Autodesk Inventor part; units mm, degrees
ref_plane "YZ Plane" through (0, 0, 0) normal (1, 0, 0) x (0, 1, 0)
ref_plane "XZ Plane" through (0, 0, 0) normal (0, 1, 0) x (-1, 0, 0)
ref_plane "XY Plane" through (0, 0, 0) normal (0, 0, 1) x (1, 0, 0)
sketch "Sketch1" plane through (0, 0, 0) normal (0, 0, 1) x (1, 0, 0)
  circle A0 centre (0, 0) radius 28.575
  circle A1 centre (0, 0) radius 19.05
  dimension "d0" = 57.15
  dimension "d8" = 38.1
sketch "Sketch2" plane through (0, 0, 0) normal (0, 0, 1) x (1, 0, 0)
  circle A0 centre (0, 0) radius 23.8125
  circle A1 centre (0, 23.8125) radius 2.5908
  circle A2 centre (-20.6222, 11.9063) radius 2.5908
  circle A3 centre (-20.6222, -11.9062) radius 2.5908
  circle A4 centre (0, -23.8125) radius 2.5908
  circle A5 centre (20.6222, -11.9063) radius 2.5908
  circle A6 centre (20.6222, 11.9062) radius 2.5908
  dimension "d15" = 47.625
  dimension "d16" = 5.1816
  dimension "d19" = 360
extrude "Extrusion1" add sketch "Sketch1" along normal blind 13.97
extrude "Extrusion2" cut sketch "Sketch2" along normal blind 13.97 contours A6 A0 | A0 A6 | A5 A0 | A0 A5 | A1 A0 | A0 A1 | A4 A0 | A0 A4 | A2 A0 | A0 A2 | A3 A0 | A0 A3
properties part number "550 Sprocket Spacer (am-0651)" material "PC/ABS Plastic"
For this review, take the finished solid that the model builds, in its own axes (mm). Give positions to 0.01 mm unless a question says otherwise; leave off trailing zeros. Write each loop counter-clockwise with the first axis right and the second up, starting at its lowest first coordinate (ties: lowest second). Pieces come first, ordered by that corner, then holes. Notation, with made-up numbers: (28.5, 64.5) -> (49.5, 64.5) arc R10 ccw to (49.5, 80.5) -> close; hole circle Ø2 at (-11, 74). An arc over 180 degrees is marked (long way). Use CSV: the item, a comma, the result in double quotes.
Q1. Mouldability with a two-part tool opening along Y and no side actions: class faces 1 (the face through (-0.562, 26.342, 6.887)), 2 (the face through (19, -6, 0)), 3 (the face through (-28.547, -1.256, 6.887)) as pulls with the +Y half, pulls with the -Y half, needs draft (parallel to the pull), parting line crosses it, or undercut.
Conclusion:
face 1,"undercut"
face 2,"needs draft"
face 3,"parting line crosses it"
Q2. To check wall thickness, follow probe 1 along Y at (x, z) = (0, 4.25) (3 decimals); probe 2 along Y at (x, z) = (-20, 11.25); probe 3 along Y at (x, z) = (23, 1.25). State the ranges of each line that lie inside material, in increasing order. Write a range as [from, to].
Conclusion:
probe 1,"[-28.575, -26.403], [-21.222, -19.05], [19.05, 21.222], [26.403, 28.575]"
probe 2,"[-20.41, -14.42], [-9.39, 9.39], [14.42, 20.41]"
probe 3,"[-16.96, -12.94], [-10.88, 10.88], [12.93, 16.96]"
Q3. Take a section at B-B, the plane y = 0. Write out the cut boundary in (x, z) (3 decimals).
Conclusion:
outline,"(-28.575, 0) -> (-19.05, 0) -> (-19.05, 13.97) -> (-28.575, 13.97) -> close; (19.05, 0) -> (28.575, 0) -> (28.575, 13.97) -> (19.05, 13.97) -> close"
Q4. Take a section at D-D, the plane z = 3.5. State how many separate pieces and enclosed holes the cut face has, then the cut area to 3 significant figures.
Conclusion:
separate pieces,"1"
enclosed holes,"7"
area,"1,300 mm2"
Q5. Take a section at C-C, the plane x = 11. Write out the cut boundary in (y, z), then the cut area to 3 significant figures.
Conclusion:
outline,"(-26.37, 0) -> (-15.55, 0) -> (-15.55, 13.97) -> (-26.37, 13.97) -> close; (15.55, 0) -> (26.37, 0) -> (26.37, 13.97) -> (15.55, 13.97) -> close"
area,"302 mm2"
Q6. Take a section at A-A, the plane x = 0. Write out the cut boundary in (y, z) (3 decimals).
Conclusion:
outline,"(-28.575, 0) -> (-26.403, 0) -> (-26.403, 13.97) -> (-28.575, 13.97) -> close; (-21.222, 0) -> (-19.05, 0) -> (-19.05, 13.97) -> (-21.222, 13.97) -> close; (19.05, 0) -> (21.222, 0) -> (21.222, 13.97) -> (19.05, 13.97) -> close; (26.403, 0) -> (28.575, 0) -> (28.575, 13.97) -> (26.403, 13.97) -> close"
Q7. For P1, Ø1, axis at x = -9, z = 11, coming from the -Y side; P2, Ø6, axis at x = 0, y = -23.81, coming from the -Z side; P3, Ø3, axis at x = -9.5, z = 5, coming from the +Y side; P4, Ø2, axis at x = 9.5, z = 8.5, coming from the +Y side, all flat-tipped, find the tip position at first contact; note any pin that passes through.
Conclusion:
P1,"y = -27.28"
P2,"z = 0"
P3,"y = 27.43"
P4,"y = 27.28"
